Part model, mm, in its own coordinate system. A direction names the side the tool comes from. Round coordinates to 2 decimals unless told otherwise and drop trailing zeros. Order: outer loops, then holes, each group sorted by start corner. A loop starts at its lowest first (then second) coordinate and runs counter-clockwise, first axis right, second up. Notation, with made-up numbers: (-20.75, -29.75) - (6.25, -29.75) arc R11 ccw to (6.25, -23.75) - close; hole circle Ø6 at (-36, 41.25). An arc over 180 degrees is marked (long way). Answer as a JSON object with one key per item and string values.
```python
from build123d import *

# Parameters (mm, degrees)
SKETCH1_W           = 24.13
SKETCH1_H           = 32.512
BOSS_EXTRUDE1_DEPTH = 1.524
SKETCH2_W           = 23.114
SKETCH2_H           = 23.114
BOSS_EXTRUDE2_DEPTH = 3.302
SKETCH5_R           = 0.889
CUT_EXTRUDE1_DEPTH  = 26.11198204


with BuildPart() as part:
    # Sketch1 → Boss-Extrude1 (new body)
    with BuildSketch(Plane(origin=(0, 0, 0), x_dir=(1, 0, 0), z_dir=(0, 1, 0))):
        Rectangle(SKETCH1_W, SKETCH1_H)
    extrude(amount=BOSS_EXTRUDE1_DEPTH)

    # Sketch2 → Boss-Extrude2 (add)
    with BuildSketch(Plane(origin=(0, 1.524, 0), x_dir=(1, 0, 0), z_dir=(0, 1, 0))):
        Rectangle(SKETCH2_W, SKETCH2_H)
    extrude(amount=BOSS_EXTRUDE2_DEPTH)

    # Sketch4 → Revolve1 (revolve)
    with BuildSketch(Plane(origin=(0, 0, 0), x_dir=(0, 0, -1), z_dir=(1, 0, 0))):
        with BuildLine():
            Line((0, 4.826), (0, 16.383))
            ThreePointArc((0, 16.383), (-8.17203307, 12.99803307), (-11.557, 4.826))
            Line((-11.557, 4.826), (0, 4.826))
        make_face()
    revolve(axis=Axis((0, 4.826, 0), (0, 1, 0)))

    # Sketch5 → Cut-Extrude1 (cut, through all)
    with BuildSketch(Plane(origin=(0, 1.524, 0), x_dir=(1, 0, 0), z_dir=(0, 1, 0))):
        with Locations(Location((0, -13.589, 0), (0, 0, 270))):
            Circle(SKETCH5_R)
        with Locations(Location((0, 13.589, 0), (0, 0, 270))):
            Circle(SKETCH5_R)
    extrude(amount=-CUT_EXTRUDE1_DEPTH, mode=Mode.SUBTRACT)


solid = part.part
```
Item 1: Cut at B-B (z = 9). Write the cut outline in (x, y) (3 decimals), plus the area to 3 significant figures.
Taken from the geometry:
{"outline": "(-12.065, 0) - (12.065, 0) - (12.065, 1.524) - (11.557, 1.524) - (11.557, 4.826) - (7.25, 4.826) arc R7.25 ccw to (-7.25, 4.826) - (-11.557, 4.826) - (-11.557, 1.524) - (-12.065, 1.524) - close", "area": "196 mm2"}
Item 2: Tool access for faces 1 (the flat face through (9, 4.826, 9)), 2 (the flat face through (9, 4.826, -9)), 3 (the flat face through (0, 3, -11.557)), 4 (the flat face through (-11.557, 3, 0)): list every direction of +Z, -Z, +X, -X, +Y, -Y with a clear straight run to the whole face (end or side of a thin tool).
Taken from the geometry:
{"face 1": "+Z, +X, +Y", "face 2": "-Z, +X, +Y", "face 3": "-Z, +X, -X, +Y", "face 4": "+Z, -Z, -X, +Y"}
Item 3: Cut at D-D (y = 14.75). Write the cut outline in (x, z).
Taken from the geometry:
{"outline": "circle Ø11.85 at (0, 0)"}
Item 4: Cut at C-C (x = 3.75). Write the cut outline in (y, z), plus the area to 3 significant figures.
Taken from the geometry:
{"outline": "(0, -16.26) - (1.52, -16.26) - (1.52, -11.56) - (4.83, -11.56) - (4.83, -10.93) arc R10.93 ccw to (4.83, 10.93) - (4.83, 11.56) - (1.52, 11.56) - (1.52, 16.26) - (0, 16.26) - close", "area": "314 mm2"}
Item 5: Cut at A-A (y = 2.75). Write the cut outline in (x, z), plus the area to 3 significant figures.
Taken from the geometry:
{"outline": "(-11.56, -11.56) - (11.56, -11.56) - (11.56, 11.56) - (-11.56, 11.56) - close", "area": "534 mm2"}
Item 6: Drop flat-ended pins along their axis: P1, Ø1, axis at x = 2.5, z = 10.5, coming from the +Y side; P2, Ø1, axis at x = 6.5, z = -3.5, coming from the -Y side; P3, Ø2.5, axis at x = -2.5, y = 4, coming from the +Z side; P4, Ø9, axis at x = -4, z = -6, coming from the +Y side. Give the stop position or say it passes through.
Taken from the geometry:
{"P1": "y = 10.08", "P2": "y = 0", "P3": "z = 11.56", "P4": "y = 16.06"}
Item 7: Two-plate mould, pull along X, no slides. Class faces 5 (the flat face through (-9, 4.826, -9)), 6 (the cylindrical face through (0.267, 0.773, 14.437)), 7 (the flat face through (12.065, 1, 0)), 8 (the cylindrical face through (0.27, 0.77, -12.74)): pulls with the +X half, pulls with the -X half, needs draft (parallel to the pull), parting line crosses it, or undercut.
Taken from the geometry:
{"face 5": "needs draft", "face 6": "undercut", "face 7": "pulls with the +X half", "face 8": "undercut"}
Item 8: Probe L1, parallel to Y at x = 10.5, z = -14; L2, parallel to Y at x = -7, z = -10.5; L3, parallel to X at y = 1.25, z = 13 (3 decimals). List the from-to ranges inside material, lowest first. Write a range as from..to.
Taken from the geometry:
{"L1": "0..1.52", "L2": "0..4.83", "L3": "-12.065..-0.666, 0.666..12.065"}
